Geometry: final body of the model. Coordinates: model frame, mm. Face numbers are marked on the shaded views. A direction names the side the tool comes from. Round coordinates to 2 decimals unless told otherwise and drop trailing zeros. Order: outer loops, then holes, each group sorted by start corner. A loop starts at its lowest first (then second) coordinate and runs counter-clockwise, first axis right, second up. Notation, with made-up numbers: M 48,50 L 91,50 A5 cw 91,58 Z; hole C 34.5,85.5 d2. An arc over 180 degrees is marked long. Put each result on its own line as item: value. Start each with the question number.
1) Section B-B, the plane y = -5. Count the separate pieces of the cut face and the enclosed holes in it, then the cut area to 3 significant figures.
2) Draft query along Y for the marked faces 5, 6 and 7. Return one class per face: pulls with the +Y half, pulls with the -Y half, needs draft (parallel to the pull), parting line crosses it, or undercut.
3) First-contact query: P1, Ø2.5, axis at y = -5, z = 11.8, coming from the +X side; P2, Ø2, axis at x = 2, y = -3, coming from the -Z side; P3, Ø2.5, axis at y = -5, z = 11.8, coming from the -X side. Flat tips, straight axial feed; report the tip coordinate or a pass-through.
4) Material intervals for probe 1 along X at (y, z) = (-7, 13.75); probe 2 along X at (y, z) = (-5.75, 12.75); probe 3 along Z at (x, y) = (-4.6, -5), sorted ascending. Write a range as [from, to].
5) Access query for the marked faces 1, 2, 3 and 4. Directions: +Z, -Z, +X, -X, +Y, -Y. A direction counts if a zero-diameter tool reaches every point of the face in a straight line with its end or side. Return the directions, or none.
6) Section A-A, the plane z = 15. Return loops of the section in (x, y), then the cut area to 3 significant figures.
from build123d import *

# Parameters (mm, degrees)
SKETCH2_R           = 1
BOSS_EXTRUDE1_DEPTH = 9
SKETCH4_W           = 3
SKETCH4_H           = 5
CUT_EXTRUDE1_DEPTH  = 15
SKETCH5_W           = 6
SKETCH5_H           = 10
CUT_EXTRUDE3_DEPTH  = 5.25
SKETCH6_R           = 1.5
CUT_EXTRUDE4_DEPTH  = 3
SKETCH7_R           = 1.5
CUT_EXTRUDE5_DEPTH  = 3


with BuildPart() as part:
    # Sketch2 → Boss-Extrude1 (new body, symmetric)
    with BuildSketch(Plane(origin=(0, 0, 0), x_dir=(0, 0, -1), z_dir=(1, 0, 0))):
        with BuildLine():
            Line((-6.491790717, 5.877052321), (-30, 0))
            add(Edge.make_bspline(
                [(-30, 0), (-30, -1.825107758), (-26.893202648, -7.805962947), (-20.772810337, -7.5), (-18.5, -7.5)],
                knots=[0, 0, 0, 0, 0.460452824, 1, 1, 1, 1], degree=3))
            Line((-18.5, -7.5), (-11.801638904, -7.5))
            ThreePointArc((-11.801638904, -7.5), (-10.647112952, -7.217446691), (-9.753559103, -6.433655861))
            Line((-9.753559103, -6.433655861), (-3.837371853, 2.018040209))
            ThreePointArc((-3.837371853, 2.018040209), (-3.825682806, 4.868506676), (-6.491790717, 5.877052321))
        make_face()
        with Locations((-11.801638904, -5)):
            Circle(SKETCH2_R, mode=Mode.SUBTRACT)
        with Locations((-5.885451655, 3.45169607)):
            Circle(SKETCH2_R, mode=Mode.SUBTRACT)
    extrude(amount=BOSS_EXTRUDE1_DEPTH, both=True)

    # Sketch4 → Cut-Extrude1 (cut)
    with BuildSketch(Plane(origin=(0, 5.95169607, 0), x_dir=(1, 0, 0), z_dir=(0, 1, 0))):
        with Locations((0, -5.885451655)):
            Rectangle(SKETCH4_W, SKETCH4_H)
    extrude(amount=-CUT_EXTRUDE1_DEPTH, mode=Mode.SUBTRACT)

    # Sketch5 → Cut-Extrude3 (cut)
    with BuildSketch(Plane.XZ.offset(7.5)):
        with Locations((0, 10.801638904)):
            Rectangle(SKETCH5_W, SKETCH5_H)
    extrude(amount=-CUT_EXTRUDE3_DEPTH, mode=Mode.SUBTRACT)

    # Sketch6 → Cut-Extrude4 (cut)
    with BuildSketch(Plane(origin=(9, 0, 0), x_dir=(0, 0, -1), z_dir=(1, 0, 0))):
        with Locations((-5.885451655, 3.45169607)):
            Circle(SKETCH6_R)
        with Locations((-11.801638904, -5)):
            Circle(SKETCH6_R)
    extrude(amount=-CUT_EXTRUDE4_DEPTH, mode=Mode.SUBTRACT)

    # Sketch7 → Cut-Extrude5 (cut)
    with BuildSketch(Plane.ZY.offset(9)):
        with Locations((5.885451655, 3.45169607)):
            Circle(SKETCH7_R)
        with Locations((11.801638904, -5)):
            Circle(SKETCH7_R)
    extrude(amount=-CUT_EXTRUDE5_DEPTH, mode=Mode.SUBTRACT)


solid = part.part
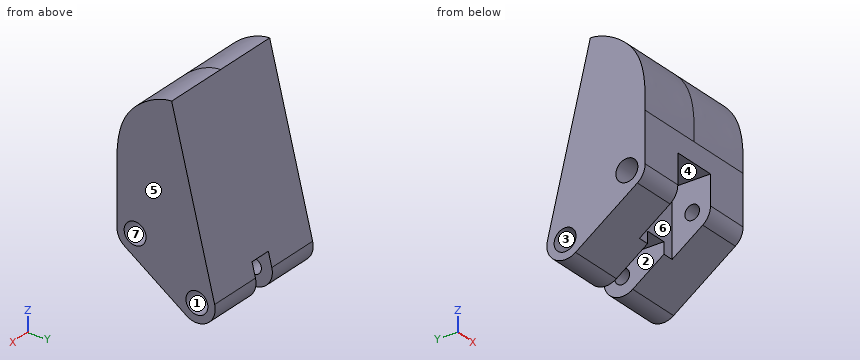
Result sheet:
1. separate pieces: 3
1. enclosed holes: 0
1. area: 268 mm2
2. face 5: needs draft
2. face 6: pulls with the -Y half
2. face 7: undercut
3. P1: stops at x = 6
3. P2: stops at z = 6.65
3. P3: stops at x = -6
4. probe 1: x = [-9, -3], [3, 9]
4. probe 2: x = [-6, -3], [3, 6]
4. probe 3: z = [8.75, 10.8], [12.8, 27.66]
5. face 1: +X
5. face 2: -Z, +Y, -Y
5. face 3: -X
5. face 4: -Z, -Y
6. outline: M -9,-7.5 L -3,-7.5 L -3,-2.25 L 3,-2.25 L 3,-7.5 L 9,-7.5 L 9,3.75 L -9,3.75 Z
6. area: 171 mm2
